from build123d import *

# Parameters (mm, degrees)
SKETCH1_R           = 9
SKETCH1_W           = 3
SKETCH1_H           = 12
BOSS_EXTRUDE1_DEPTH = 3
SKETCH2_R           = 1.5
CUT_EXTRUDE1_DEPTH  = 139.166566144


with BuildPart() as part:
    # Sketch1 → Boss-Extrude1 (new body)
    with BuildSketch(Plane(origin=(0, 0, 0), x_dir=(1, 0, 0), z_dir=(0, 1, 0))):
        with BuildLine():
            Line((50, -81), (50, 11))
            Line((50, 11), (48.5, 11))
            Line((48.5, 11), (48.5, 23))
            Line((48.5, 23), (50, 23))
            Line((50, 23), (50, 81))
            Line((50, 81), (75, 81))
            ThreePointArc((75, 81), (0, 116), (-75, 81))
            Line((-75, 81), (-50, 81))
            Line((-50, 81), (-50, 23))
            Line((-50, 23), (-48.5, 23))
            Line((-48.5, 23), (-48.5, 11))
            Line((-48.5, 11), (-50, 11))
            Line((-50, 11), (-50, -81))
            ThreePointArc((-50, -81), (0, -91.912878854), (50, -81))
        make_face()
        with Locations(Location((0, 81, 0), (0, 0, 270))):
            Circle(SKETCH1_R, mode=Mode.SUBTRACT)
        with Locations((-29, 17)):
            Rectangle(SKETCH1_W, SKETCH1_H, mode=Mode.SUBTRACT)
        with Locations((29, 17)):
            Rectangle(SKETCH1_W, SKETCH1_H, mode=Mode.SUBTRACT)
        with BuildLine():
            ThreePointArc((31.93002338, 105.869875383), (0, 111.5), (-31.93002338, 105.869875383))
            ThreePointArc((-31.93002338, 105.869875383), (-32.826532097, 103.947306237), (-30.90396295, 103.050797521))
            ThreePointArc((-30.90396295, 103.050797521), (0, 108.5), (30.90396295, 103.050797521))
            ThreePointArc((30.90396295, 103.050797521), (32.826532097, 103.947306237), (31.93002338, 105.869875383))
        make_face(mode=Mode.SUBTRACT)
    extrude(amount=BOSS_EXTRUDE1_DEPTH)

    # Sketch2 → Cut-Extrude1 (cut, through all)
    with BuildSketch(Plane(origin=(0, 3, 0), x_dir=(1, 0, 0), z_dir=(0, 1, 0))):
        with Locations(Location((15, -60, 0), (0, 0, 270))):
            Circle(SKETCH2_R)
        with Locations(Location((15, -85, 0), (0, 0, 270))):
            Circle(SKETCH2_R)
        with Locations(Location((-15, -85, 0), (0, 0, 90))):
            Circle(SKETCH2_R)
        with Locations(Location((-15, -60, 0), (0, 0, 90))):
            Circle(SKETCH2_R)
    extrude(amount=-CUT_EXTRUDE1_DEPTH, mode=Mode.SUBTRACT)


solid = part.part
Can you work these out from the model? Positions are in its coordinate system, mm. A direction names the side the tool comes from. Round coordinates to 2 decimals unless told otherwise and drop trailing zeros. Order: outer loops, then holes, each group sorted by start corner. A loop starts at its lowest first (then second) coordinate and runs counter-clockwise, first axis right, second up. Notation, with made-up numbers: (-37, 79) -> (-27, 79) arc R13 ccw to (-27, 84) -> close; hole circle Ø4 at (-9, 9.5). An arc over 180 degrees is marked (long way). Write each question's results on one line, items separated by ' | '. Start each with the question number.
Item 1: If we section it at C-C, the plane z = -87: Write out the boundary of the cut face in (x, y).
Item 2: Please list where these lines run through material, in increasing order: L1, parallel to X at y = 1.3, z = 60; L2, parallel to X at y = 2.15, z = 3.5; L3, parallel to Z at x = 30, y = 2.
Item 3: If we section it at A-A, the plane x = 0: Write out the boundary of the cut face in (y, z), then the cut area to 3 significant figures.
Item 4: Thinking about a two-plate mould opening in X: for faces 3 (the cylindrical face through (1.196, 1.479, -115.993)), 4 (the flat face through (-1, 3, -13)), 5 (the cylindrical face through (2.703, 1.479, -72.416)), which applies, +X half, -X half, draft (parallel to the pull), parting line (faces both ways), or undercut?
Item 5: Will these pins go through, and if not, where does the flat tip stop? pin 1 (1.5 mm diameter, centred on x = 29, y = 1, fed in from +Z); pin 2 (1.5 mm diameter, centred on y = 2, z = -20, fed in from -X); pin 3 (1.6 mm diameter, centred on x = -49.5, y = 2, fed in from -Z).
Item 6: If we section it at D-D, the plane z = -38.5: Write out the boundary of the cut face in (x, y).
Item 7: If we section it at B-B, the plane y = 1.6: State how many separate pieces and enclosed holes the cut face has, then the cut area to 3 significant figures.
Item 8: Which directions (+Z, -Z, +X, -X, +Y, -Y) give clear straight access to the entire face, cutting with the end or side of a thin tool? Please do faces 1 (the cylindrical face through (0.5, 1.5, -111.5)), 2 (the flat face through (-1, 0, -13)).
Results:
1) outline: (-69.53, 0) -> (-6.71, 0) -> (-6.71, 3) -> (-69.53, 3) -> close; (6.71, 0) -> (69.53, 0) -> (69.53, 3) -> (6.71, 3) -> close
2) L1: x = -50 to -16.5, -13.5 to 13.5, 16.5 to 50 | L2: x = -50 to 50 | L3: z = -111.29 to -106.55, -103.37 to -23, -11 to 88.1
3) outline: (0, -116) -> (3, -116) -> (3, -111.5) -> (0, -111.5) -> close; (0, -108.5) -> (3, -108.5) -> (3, -90) -> (0, -90) -> close; (0, -72) -> (3, -72) -> (3, 91.91) -> (0, 91.91) -> close | area: 561 mm2
4) face 3: parting line | face 4: draft | face 5: undercut
5) pin 1: stops at z = 88.54 | pin 2: stops at x = -48.5 | pin 3: stops at z = -103.02
6) outline: (-50, 0) -> (50, 0) -> (50, 3) -> (-50, 3) -> close
7) separate pieces: 1 | enclosed holes: 8 | area: 20,000 mm2
8) face 1: +Y, -Y | face 2: +Z, -Z, +X, -X, -Y
